```python
from build123d import *

# Parameters (mm, degrees)
SKETCH1_W           = 40
SKETCH1_H           = 40
BOSS_EXTRUDE1_DEPTH = 40
SKETCH2_W           = 10
SKETCH2_H           = 10
CUT_EXTRUDE1_DEPTH  = 40
SKETCH3_W           = 10
SKETCH3_H           = 10
CUT_EXTRUDE2_DEPTH  = 20
SKETCH5_W           = 10
SKETCH5_H           = 10
CUT_EXTRUDE3_DEPTH  = 20
CUT_EXTRUDE5_DEPTH  = 30
CUT_EXTRUDE6_DEPTH  = 10


with BuildPart() as part:
    # Sketch1 → Boss-Extrude1 (new body)
    with BuildSketch(Plane.XY):
        with Locations((20, 20)):
            Rectangle(SKETCH1_W, SKETCH1_H)
    extrude(amount=BOSS_EXTRUDE1_DEPTH)

    # Sketch2 → Cut-Extrude1 (cut)
    with BuildSketch(Plane.ZY):
        with Locations((25, 35)):
            Rectangle(SKETCH2_W, SKETCH2_H)
        Polygon((40, 10), (40, 40), (30, 40), (30, 30), (30, 10), align=None)
    extrude(amount=-CUT_EXTRUDE1_DEPTH, mode=Mode.SUBTRACT)

    # Sketch3 → Cut-Extrude2 (cut)
    with BuildSketch(Plane(origin=(0, 30, 0), x_dir=(1, 0, 0), z_dir=(0, 1, 0))):
        with Locations((35, -25)):
            Rectangle(SKETCH3_W, SKETCH3_H)
    extrude(amount=-CUT_EXTRUDE2_DEPTH, mode=Mode.SUBTRACT)

    # Sketch5 → Cut-Extrude3 (cut)
    with BuildSketch(Plane(origin=(0, 30, 0), x_dir=(1, 0, 0), z_dir=(0, 1, 0))):
        with Locations((5, -25)):
            Rectangle(SKETCH5_W, SKETCH5_H)
    extrude(amount=-CUT_EXTRUDE3_DEPTH, mode=Mode.SUBTRACT)

    # Sketch6 → Cut-Extrude5 (cut)
    with BuildSketch(Plane(origin=(0, 40, 0), x_dir=(1, 0, 0), z_dir=(0, 1, 0))):
        Polygon((10, -20), (0, 0), (0, -20), align=None)
    extrude(amount=-CUT_EXTRUDE5_DEPTH, mode=Mode.SUBTRACT)

    # Sketch7 → Cut-Extrude6 (cut)
    with BuildSketch(Plane.XY.offset(30)):
        Polygon((10, 30), (30, 10), (30, 30), align=None)
    extrude(amount=-CUT_EXTRUDE6_DEPTH, mode=Mode.SUBTRACT)


solid = part.part
```
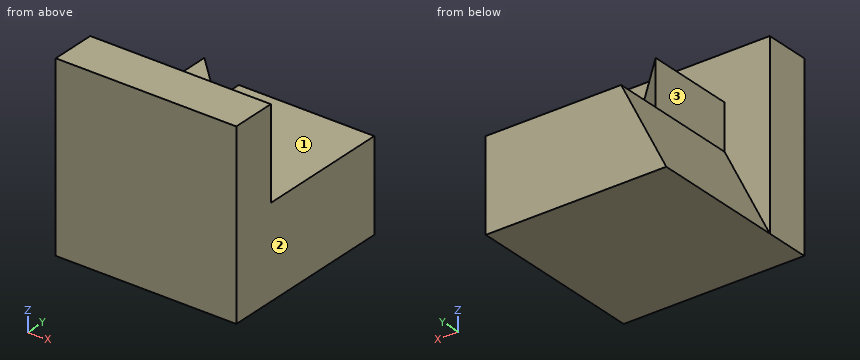
Design review of the part built by this model. Coordinates are the model's own, in mm. Face numbers are marked on the shaded views. A direction names the side the tool comes from. Give positions to 0.01 mm unless a question says otherwise; leave off trailing zeros. Write each loop counter-clockwise with the first axis right and the second up, starting at its lowest first coordinate (ties: lowest second). Pieces come first, ordered by that corner, then holes. Notation, with made-up numbers: (86, 86.5) -> (109, 86.5) arc R18 ccw to (109, 116.5) -> close; hole circle Ø6 at (70, 30). An arc over 180 degrees is marked (long way). Answer in a Markdown table with one row per item.
(1) To check wall thickness, follow probe 1 along Y at (x, z) = (35, 31); probe 2 along Z at (x, y) = (30, 21); probe 3 along Z at (x, y) = (16.5, 16.5). State the ranges of each line that lie inside material, in increasing order.
Results:
| item | result |
|---|---|
| probe 1 | 0 to 10 |
| probe 2 | 0 to 20 |
| probe 3 | 0 to 30 |
(2) Consider section B-B (z = 27). State the section outline as (x, y) points.
Results:
| item | result |
|---|---|
| outline | (0, 0) -> (40, 0) -> (40, 10) -> (30, 10) -> (10, 30) -> (10, 10) -> (0, 10) -> close |
(3) Consider section D-D (x = 14.5). State the section outline as (y, z) points.
Results:
| item | result |
|---|---|
| outline | (0, 0) -> (40, 0) -> (40, 20) -> (25.5, 20) -> (25.5, 30) -> (10, 30) -> (10, 40) -> (0, 40) -> close |
(4) Clearance check with flat-ended pins moving along their axes: pin 1 (1 mm diameter, centred on y = 35, z = 10.5, fed in from -X); pin 2 (2 mm diameter, centred on x = 18, y = 11.5, fed in from +Z); pin 3 (15 mm diameter, centred on x = 25.5, y = 29.5, fed in from +Z). State where each tip first meets the part, or that it passes through.
Results:
| item | result |
|---|---|
| pin 1 | x = 5 |
| pin 2 | z = 30 |
| pin 3 | z = 20 |
(5) For the marked faces 1, 2 and 3, list the 3-axis set-ups (+Z, -Z, +X, -X, +Y, -Y) from which the entire face can be reached by the end or side of a thin tool; tool diameter is ignored.
Results:
| item | result |
|---|---|
| face 1 | +Z, +X, +Y |
| face 2 | +Z, -Z, +X, +Y, -Y |
| face 3 | +Z, -X, +Y |
(6) Consider section C-C (y = 28). State the section outline as (x, z) points.
Results:
| item | result |
|---|---|
| outline | (0, 0) -> (40, 0) -> (40, 20) -> (12, 20) -> (12, 30) -> (10, 30) -> (10, 20) -> close |
(7) Consider section A-A (x = 19.5). State the section outline as (y, z) points, then the cut area to 4 significant figures.
Results:
| item | result |
|---|---|
| outline | (0, 0) -> (40, 0) -> (40, 20) -> (20.5, 20) -> (20.5, 30) -> (10, 30) -> (10, 40) -> (0, 40) -> close |
| area | 1,105 mm2 |
